CAD build for the part. Positions are in the model's coordinates, mm. A direction names the side the tool comes from. Round coordinates to 2 decimals unless told otherwise and drop trailing zeros. Write each loop counter-clockwise with the first axis right and the second up, starting at its lowest first coordinate (ties: lowest second). Pieces come first, ordered by that corner, then holes. Notation, with made-up numbers: (88, 23.25) - (130, 23.25) arc R24 cw to (130, 42.25) - close; hole circle Ø7 at (26.25, 58). An arc over 180 degrees is marked (long way). Use one line per item in the form item = value. Start each with the question number.
Item 1: Pull direction X, two halves, no side cores. Call faces 1 (the flat face through (38, 31, 2.54)), 2 (the cylindrical face through (63.143, 14.979, 4.418)), 3 (the cylindrical face through (74.672, 62.051, 4.472)): +X half, -X half, draft (parallel to the pull), parting line (faces both ways), or undercut.
Item 2: Drill centre lines: L1, parallel to Y at x = 59, z = 5.25; L2, parallel to X at y = 13, z = 3.5; L3, parallel to Z at x = 22, y = 47.5. Where is each one in solid material? Low to high.
Item 3: Tool access for faces 4 (the flat face through (3, 19.05, 1)), 5 (the flat face through (19.05, 3, 1)), 6 (the flat face through (6.35, 12, 1)): list every direction of +Z, -Z, +X, -X, +Y, -Y with a clear straight run to the whole face (end or side of a thin tool).
Item 4: Band-saw the part on C-C, the plane x = 60.5. List the corners of the cut face in (y, z), and give its area (3 significant figures).
Item 5: Band-saw the part on D-D, the plane y = 25.5. List the corners of the cut face in (x, z), and give its area (3 significant figures).
Item 6: Band-saw the part on B-B, the plane z = 1.5. List the corners of the cut face in (x, y).
Item 7: Band-saw the part on A-A, the plane y = 55. List the corners of the cut face in (x, z).
Item 8: Pin check, flat tips, straight feed: pin 1 (5.5 mm diameter, centred on x = 58.62, y = 13.56, fed in from +Z); pin 2 (12 mm diameter, centred on x = 58.98, y = 51.93, fed in from -Z); pin 3 (1.3 mm diameter, centred on x = 2.5, z = 1, fed in from +Y); pin 4 (0.8 mm diameter, centred on y = 3.5, z = 1, fed in from +X). Stop position of each tip, or through.
from build123d import *

# Parameters (mm, degrees)
F0_W     = 76.2
F0_H     = 63.5
F0_R     = 3.5209789872
F0_R_2   = 4.7369922421
F0_R_3   = 4.4117780633
F0_R_4   = 4.6311273859
F1_DEPTH = 6.35
F3_DEPTH = 2.54
F4_R     = 5.08
F5_R     = 1.27


with BuildPart() as f1:
    # F0 (on Top) → F1 (new body)
    with BuildSketch(Plane.XY):
        with Locations((38.1, 31.75)):
            Rectangle(F0_W, F0_H)
        with Locations((17.7809670568, 14.9641726166)):
            Circle(F0_R, mode=Mode.SUBTRACT)
        with Locations((58.6243532598, 13.5557809845)):
            Circle(F0_R_2, mode=Mode.SUBTRACT)
        with Locations((39.2589494586, 23.7666256726)):
            Circle(F0_R_3, mode=Mode.SUBTRACT)
        with Locations((58.9764490724, 51.9344769418)):
            Circle(F0_R_4, mode=Mode.SUBTRACT)
    extrude(amount=F1_DEPTH)

    # F2 (on face) → F3 (cut)
    with BuildSketch(Plane(origin=(0, 0, 0), x_dir=(1, 0, 0), z_dir=(0, 0, -1))):
        Polygon((19.05, -6.3181049854), (6.3500011563, -6.3181049854), (6.3500011563, -19.05), (0, -19.05), (0, -63.5), (76.2, -63.5), (76.2, 0), (19.05, 0), align=None)
    extrude(amount=-F3_DEPTH, mode=Mode.SUBTRACT)

    # F4
    f4_edges = [f1.edges().sort_by_distance(p)[0] for p in [
        (0, 63.5, 4.445),
        (76.2, 63.5, 4.445),
        (76.2, 0, 4.445),
        (0, 0, 3.175),
    ]]
    fillet(f4_edges, radius=F4_R)

    # F5
    f5_edges = [f1.edges().sort_by_distance(p)[0] for p in [
        (6.350001, 19.05, 1.27),
        (19.05, 6.318105, 1.27),
        (0, 19.05, 1.27),
        (19.05, 0, 1.27),
    ]]
    fillet(f5_edges, radius=F5_R)


solid = f1.part
Determined:
q1.face_1 = draft
q1.face_2 = undercut
q1.face_3 = +X half
q2.L1 = 0 to 8.83, 18.28 to 47.3, 56.57 to 63.5
q2.L2 = 0 to 14.86, 20.7 to 53.92, 63.33 to 76.2
q2.L3 = 2.54 to 6.35
q3.face_4 = -Z, +X, -X, +Y
q3.face_5 = -Z, +X, +Y, -Y
q3.face_6 = -Z, +X, +Y
q4.outline = (0, 2.54) - (9.21, 2.54) - (9.21, 6.35) - (0, 6.35) - close; (17.91, 2.54) - (47.56, 2.54) - (47.56, 6.35) - (17.91, 6.35) - close; (56.31, 2.54) - (63.5, 2.54) - (63.5, 6.35) - (56.31, 6.35) - close
q4.area = 175 mm²
q5.outline = (0, 2.54) - (35.2, 2.54) - (35.2, 6.35) - (0, 6.35) - close; (43.32, 2.54) - (76.2, 2.54) - (76.2, 6.35) - (43.32, 6.35) - close
q5.area = 259 mm²
q6.outline = (0, 5.08) arc R5.08 ccw to (5.08, 0) - (17.78, 0) arc R1.27 ccw to (19.05, 1.27) - (19.05, 5.05) arc R1.27 ccw to (17.78, 6.32) - (6.35, 6.32) - (6.35, 17.78) arc R1.27 ccw to (5.08, 19.05) - (1.27, 19.05) arc R1.27 ccw to (0, 17.78) - close
q7.outline = (0, 2.54) - (55.51, 2.54) - (55.51, 6.35) - (0, 6.35) - close; (62.45, 2.54) - (76.2, 2.54) - (76.2, 6.35) - (62.45, 6.35) - close
q8.pin_1 = through
q8.pin_2 = 2.54
q8.pin_3 = 19.05
q8.pin_4 = 19.05
